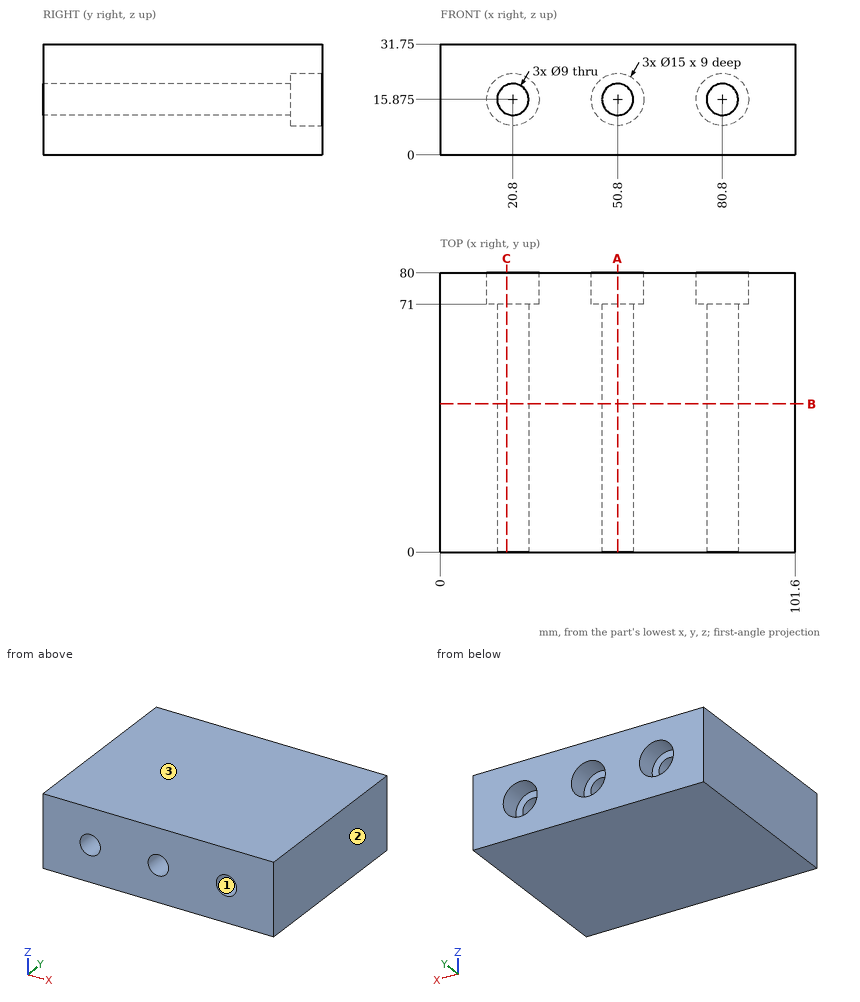
Geometry: see drawing. Coordinates: mm, zero at the bounding-box minimum. Coordinates: 2 decimals unless noted, no trailing zeros. Order: outer loops, then holes, each group sorted by start corner. A loop starts at its lowest first (then second) coordinate and runs counter-clockwise, first axis right, second up. Notation, with made-up numbers: M -27.5,55 L -10.5,55 A24 cw -10.5,76 Z; hole C 82,23 d6. An arc over 180 degrees is marked long. Write each question's results on one line, items separated by ' | '. Start each with the question number.
1) Line query: line 1 (X direction, y = 73.5, z = 14.5); line 2 (Z direction, x = 50, y = 75); line 3 (Z direction, x = 81.5, y = 37). Output: solid intervals per line, ascending. Write a range as from..to.
2) Draft query along Z for the marked faces 1, 2 and 3. Return one class per face: released by +Z, released by -Z, zero draft, split by the parting line, or undercut.
3) Contact query for flat-ended pins moving along their axis: pin 1 Ø10 at (y, z) = (28, 20) entering from -X; pin 2 Ø10.5 at (x, z) = (50.8, 15.875) entering from +Y. Output: stop coordinate, or through.
4) Section query A-A (x = 50.8). Return the cut outline in (y, z) (3 decimals).
5) Section query B-B (y = 42.5). Return the cut outline in (x, z) (3 decimals), plus the area to 3 significant figures.
6) Section query C-C (x = 19). Return the cut outline in (y, z), plus the area to 3 significant figures.
Answers:
1) line 1: x = 0..13.43, 28.17..43.43, 58.17..73.43, 88.17..101.6 | line 2: z = 0..8.42, 23.33..31.75 | line 3: z = 0..11.43, 20.32..31.75
2) face 1: undercut | face 2: zero draft | face 3: released by +Z
3) pin 1: stops at x = 0 | pin 2: stops at y = 71
4) outline: M 0,0 L 80,0 L 80,8.375 L 71,8.375 L 71,11.375 L 0,11.375 Z; M 0,20.375 L 71,20.375 L 71,23.375 L 80,23.375 L 80,31.75 L 0,31.75 Z
5) outline: M 0,0 L 101.6,0 L 101.6,31.75 L 0,31.75 Z; hole C 20.8,15.875 d9; hole C 50.8,15.875 d9; hole C 80.8,15.875 d9 | area: 3,030 mm^2
6) outline: M 0,0 L 80,0 L 80,8.59 L 71,8.59 L 71,11.75 L 0,11.75 Z; M 0,20 L 71,20 L 71,23.16 L 80,23.16 L 80,31.75 L 0,31.75 Z | area: 1,820 mm^2
